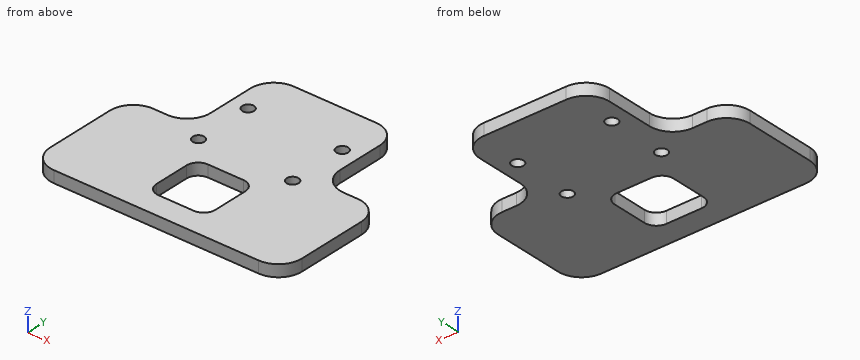
from build123d import *

# Parameters (mm, degrees)
SKETCH1_4_R         = 2.5
SKETCH1_4_W         = 25
SKETCH1_4_H         = 25
BOSS_EXTRUDE2_DEPTH = 5
FILLET3_R           = 10
FILLET4_R           = 5


with BuildPart() as part:
    # Sketch1_4 → Boss-Extrude2 (new body)
    with BuildSketch(Plane.XY):
        Polygon((-53.5, -25), (53.5, -25), (53.5, 25), (27.5, 25), (27.5, 65), (-27.5, 65), (-27.5, 25), (-53.5, 25), align=None)
        with Locations((-20, 45)):
            Circle(SKETCH1_4_R, mode=Mode.SUBTRACT)
        with Locations((-20, 20)):
            Circle(SKETCH1_4_R, mode=Mode.SUBTRACT)
        with Locations((20, 20)):
            Circle(SKETCH1_4_R, mode=Mode.SUBTRACT)
        with Locations((20, 45)):
            Circle(SKETCH1_4_R, mode=Mode.SUBTRACT)
        with Locations((0, -2.5)):
            Rectangle(SKETCH1_4_W, SKETCH1_4_H, mode=Mode.SUBTRACT)
    extrude(amount=BOSS_EXTRUDE2_DEPTH)

    # Fillet3
    fillet3_edges = [part.edges().sort_by_distance(p)[0] for p in [
        (-27.5, 65, 2.5),
        (27.5, 65, 2.5),
        (27.5, 25, 2.5),
        (53.5, 25, 2.5),
        (53.5, -25, 2.5),
        (-53.5, -25, 2.5),
        (-53.5, 25, 2.5),
        (-27.5, 25, 2.5),
    ]]
    fillet(fillet3_edges, radius=FILLET3_R)

    # Fillet4
    fillet4_edges = [part.edges().sort_by_distance(p)[0] for p in [
        (12.5, 10, 2.5),
        (-12.5, 10, 2.5),
        (-12.5, -15, 2.5),
        (12.5, -15, 2.5),
    ]]
    fillet(fillet4_edges, radius=FILLET4_R)


solid = part.part
Geometry: final body of the model. Coordinates: model frame, mm. Coordinates: 2 decimals unless noted, no trailing zeros. Order: outer loops, then holes, each group sorted by start corner. A loop starts at its lowest first (then second) coordinate and runs counter-clockwise, first axis right, second up. Notation, with made-up numbers: M 22,22.25 L 81,22.25 A18 ccw 81,33.25 Z; hole C 50.25,28 d4. An arc over 180 degrees is marked long. One line per question, with ' | ' between items. Start each with the question number.
Item 1: Ray query, probe 1 along Y at (x, z) = (-7.5, 2.95); probe 2 along Y at (x, z) = (20, 1.25); probe 3 along X at (y, z) = (-10.5, 2.35). Return the intervals inside material, ascending. Write a range as [from, to].
Item 2: Cut plane A-A, the plane y = 45. Return the cut outline in (x, z).
Item 3: Cut plane C-C, the plane x = 20. Return the cut outline in (y, z), then the cut area to 3 significant figures.
Item 4: Cut plane D-D, the plane y = -4. Return the cut outline in (x, z), then the cut area to 3 significant figures.
Item 5: Pin query (flat end, axial travel): pin 1 Ø2.5 at (y, z) = (41.5, 2) entering from -X; pin 2 Ø1.5 at (x, z) = (-39, 3) entering from +Y; pin 3 Ø6 at (x, y) = (-20, 20) entering from +Z. Return the tip coordinate at first contact, or that it passes through.
Item 6: Cut plane B-B, the plane z = 2.2. Return the cut outline in (x, y).
A:
1) probe 1: y = [-25, -15], [10, 65] | probe 2: y = [-25, 17.5], [22.5, 42.5], [47.5, 64.68] | probe 3: x = [-53.5, -12.47], [12.47, 53.5]
2) outline: M -27.5,0 L -22.5,0 L -22.5,5 L -27.5,5 Z; M -17.5,0 L 17.5,0 L 17.5,5 L -17.5,5 Z; M 22.5,0 L 27.5,0 L 27.5,5 L 22.5,5 Z
3) outline: M -25,0 L 17.5,0 L 17.5,5 L -25,5 Z; M 22.5,0 L 42.5,0 L 42.5,5 L 22.5,5 Z; M 47.5,0 L 64.68,0 L 64.68,5 L 47.5,5 Z | area: 398 mm2
4) outline: M -53.5,0 L -12.5,0 L -12.5,5 L -53.5,5 Z; M 12.5,0 L 53.5,0 L 53.5,5 L 12.5,5 Z | area: 410 mm2
5) pin 1: stops at x = -27.5 | pin 2: stops at y = 25 | pin 3: stops at z = 5
6) outline: M -53.5,-15 A10 ccw -43.5,-25 L 43.5,-25 A10 ccw 53.5,-15 L 53.5,15 A10 ccw 43.5,25 L 37.5,25 A10 cw 27.5,35 L 27.5,55 A10 ccw 17.5,65 L -17.5,65 A10 ccw -27.5,55 L -27.5,35 A10 cw -37.5,25 L -43.5,25 A10 ccw -53.5,15 Z; hole C -20,20 d5; hole C -20,45 d5; hole M -12.5,-10 A5 ccw -7.5,-15 L 7.5,-15 A5 ccw 12.5,-10 L 12.5,5 A5 ccw 7.5,10 L -7.5,10 A5 ccw -12.5,5 Z; hole C 20,20 d5; hole C 20,45 d5
